```python
from build123d import *

# Parameters (mm, degrees)
F0_R     = 12.5
F0_R_2   = 8
F1_DEPTH = 2.5
F3_DEPTH = 5
F4_SIZE  = 0.5


with BuildPart() as f1:
    # F0 (on Top) → F1 (new body, symmetric)
    with BuildSketch(Plane.XY):
        Circle(F0_R)
        Circle(F0_R_2, mode=Mode.SUBTRACT)
    extrude(amount=F1_DEPTH, both=True)

    # F2 (on face) → F3 (join)
    with BuildSketch(Plane.XY.offset(2.5)):
        with BuildLine():
            ThreePointArc((-4.9102540378, 11.4951905284), (-2.5060046284, 12.2462214908), (0, 12.5))
            Line((0, 12.5), (0, 20))
            Line((0, 20), (-4.9102540378, 11.4951905284))
        make_face()
        with BuildLine():
            Line((0, 20), (0, 12.5))
            ThreePointArc((0, 12.5), (2.5060046284, 12.2462214908), (4.9102540378, 11.4951905284))
            Line((4.9102540378, 11.4951905284), (0, 20))
        make_face()
        with BuildLine():
            Line((17.3205080757, 10), (7.5, 10))
            ThreePointArc((7.5, 10), (10.8253175473, 6.25), (12.4102540378, 1.4951905284))
            Line((12.4102540378, 1.4951905284), (17.3205080757, 10))
        make_face()
        with BuildLine():
            ThreePointArc((-12.4102540378, 1.4951905284), (-10.8253175473, 6.25), (-7.5, 10))
            Line((-7.5, 10), (-17.3205080757, 10))
            Line((-17.3205080757, 10), (-12.4102540378, 1.4951905284))
        make_face()
        with BuildLine():
            ThreePointArc((-7.5, -10), (-10.8253175473, -6.25), (-12.4102540378, -1.4951905284))
            Line((-12.4102540378, -1.4951905284), (-17.3205080757, -10))
            Line((-17.3205080757, -10), (-7.5, -10))
        make_face()
        with BuildLine():
            Line((17.3205080757, -10), (12.4102540378, -1.4951905284))
            ThreePointArc((12.4102540378, -1.4951905284), (10.8253175473, -6.25), (7.5, -10))
            Line((7.5, -10), (17.3205080757, -10))
        make_face()
        with BuildLine():
            ThreePointArc((4.9102540378, -11.4951905284), (0, -12.5), (-4.9102540378, -11.4951905284))
            Line((-4.9102540378, -11.4951905284), (0, -20))
            Line((0, -20), (4.9102540378, -11.4951905284))
        make_face()
    extrude(amount=-F3_DEPTH)

    # F4
    f4_edges = [f1.edges().sort_by_distance(p)[0] for p in [
        (12.5, 0, 2.5),
        (14.865381, 5.747595, 2.5),
        (12.410254, 10, 2.5),
        (6.25, 10.825318, 2.5),
        (2.455127, 15.747595, 2.5),
        (-2.455127, 15.747595, 2.5),
        (-6.25, 10.825318, 2.5),
        (-12.410254, 10, 2.5),
        (-14.865381, 5.747595, 2.5),
        (-12.5, 0, 2.5),
        (-14.865381, -5.747595, 2.5),
        (-12.410254, -10, 2.5),
        (-6.25, -10.825318, 2.5),
        (-2.455127, -15.747595, 2.5),
        (2.455127, -15.747595, 2.5),
        (6.25, -10.825318, 2.5),
        (12.410254, -10, 2.5),
        (14.865381, -5.747595, 2.5),
        (-8, 0, 2.5),
        (14.865381, 5.747595, -2.5),
        (12.410254, 10, -2.5),
        (6.25, 10.825318, -2.5),
        (2.455127, 15.747595, -2.5),
        (-2.455127, 15.747595, -2.5),
        (-6.25, 10.825318, -2.5),
        (-12.410254, 10, -2.5),
        (-14.865381, 5.747595, -2.5),
        (-12.5, 0, -2.5),
        (-14.865381, -5.747595, -2.5),
        (-12.410254, -10, -2.5),
        (-6.25, -10.825318, -2.5),
        (-2.455127, -15.747595, -2.5),
        (2.455127, -15.747595, -2.5),
        (6.25, -10.825318, -2.5),
        (12.410254, -10, -2.5),
        (14.865381, -5.747595, -2.5),
        (12.5, 0, -2.5),
        (-8, 0, -2.5),
    ]]
    chamfer(f4_edges, length=F4_SIZE)


solid = f1.part
```
Geometry: final body of the model. Coordinates: model frame, mm. A direction names the side the tool comes from. Round coordinates to 2 decimals unless told otherwise and drop trailing zeros. Loops run counter-clockwise (first coordinate to the right, second up) from the corner with the lowest first, then second, coordinate; pieces in that order, holes last.
Item 1: Contact query for flat-ended pins moving along their axis: P1, Ø2, axis at x = 12.5, z = 0.5, coming from the +Y side; P2, Ø3, axis at x = 2, z = -0.5, coming from the -Y side; P3, Ø1.2, axis at x = -10.5, z = 0.5, coming from the -Y side. Output: stop coordinate, or through.
Checked values:
P1: stops at y = 10
P2: stops at y = -19.13
P3: stops at y = -10
Item 2: Reachability of faces 5 (the flat face through (-14.9, 5.81, 0.03)), 6 (the flat face through (14.64, -5.86, 2.25)), 7 (the flat face through (-12, -10, 0)) from +Z, -Z, +X, -X, +Y, -Y: full face, straight path, thin tool, end or side. Return the list, or none.
Checked values:
face 5: +Z, -Z, -X
face 6: +Z, +X
face 7: +Z, -Z, -X, -Y
Item 3: Mould query, pull axis Y, two halves, no side actions, for faces 1 (the flat face through (-2.313, -15.487, 2.254)), 2 (the flat face through (14.83, 5.69, 0.03)), 3 (the flat face through (-14.64, 5.86, 2.25)), 4 (the flat face through (2.49, 15.69, 0.03)). Classes: released by +Y, released by -Y, zero draft, split by the parting line, or undercut.
Checked values:
face 1: released by -Y
face 2: undercut
face 3: undercut
face 4: released by +Y
Item 4: Section C-C, the plane x = -9. Output: boundary loops of the cut face in (y, z), plus the area to 3 significant figures.
Checked values:
outline: (-10, -2) - (-9.5, -2.5) - (9.5, -2.5) - (10, -2) - (10, 2) - (9.5, 2.5) - (-9.5, 2.5) - (-10, 2) - close
area: 99.5 mm2
Item 5: Line query: L1, parallel to X at y = -2, z = -0.5; L2, parallel to X at y = 5.5, z = 2.2; L3, parallel to Y at x = -7.5, z = 2.3. Output: solid intervals per line, ascending.
Checked values:
L1: x = -12.7 to -7.75, 7.75 to 12.7
L2: x = -14.49 to -6.08, 6.08 to 14.49
L3: y = -9.7 to -3.56, 3.56 to 9.7
Item 6: Section B-B, the plane y = 0. Output: boundary loops of the cut face in (x, z), plus the area to 3 significant figures.
Checked values:
outline: (-12.5, -2) - (-12, -2.5) - (-8.5, -2.5) - (-8, -2) - (-8, 2) - (-8.5, 2.5) - (-12, 2.5) - (-12.5, 2) - close; (8, -2) - (8.5, -2.5) - (12, -2.5) - (12.5, -2) - (12.5, 2) - (12, 2.5) - (8.5, 2.5) - (8, 2) - close
area: 44.0 mm2
Item 7: Section D-D, the plane x = -15. Output: boundary loops of the cut face in (y, z), plus the area to 3 significant figures.
Checked values:
outline: (-10, -2) - (-9.5, -2.5) - (-6.98, -2.5) - (-5.98, -2) - (-5.98, 2) - (-6.98, 2.5) - (-9.5, 2.5) - (-10, 2) - close; (5.98, -2) - (6.98, -2.5) - (9.5, -2.5) - (10, -2) - (10, 2) - (9.5, 2.5) - (6.98, 2.5) - (5.98, 2) - close
area: 38.7 mm2
Item 8: Section A-A, the plane z = 0.05. Output: boundary loops of the cut face in (x, y), plus the area to 3 significant figures.
Checked values:
outline: (-17.32, -10) - (-7.5, -10) arc R12.5 ccw to (-4.91, -11.5) - (0, -20) - (4.91, -11.5) arc R12.5 ccw to (7.5, -10) - (17.32, -10) - (12.41, -1.5) arc R12.5 ccw to (12.41, 1.5) - (17.32, 10) - (7.5, 10) arc R12.5 ccw to (4.91, 11.5) - (0, 20) - (-4.91, 11.5) arc R12.5 ccw to (-7.5, 10) - (-17.32, 10) - (-12.41, 1.5) arc R12.5 ccw to (-12.41, -1.5) - close; hole circle Ø16 at (0, 0)
area: 501 mm2
